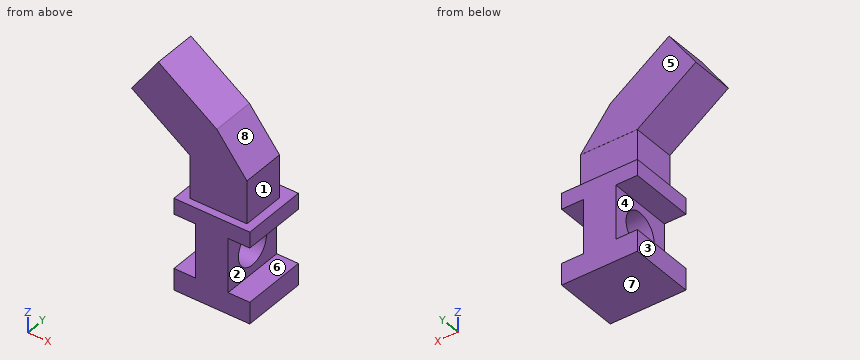
```python
from build123d import *

# Parameters (mm, degrees)
F1_DEPTH = 76.2
F2_R     = 21.9538330402
F3_DEPTH = 63.501
F4_W     = 66.6200816631
F4_H     = 50.9327836335
F5_DEPTH = 50.292
F7_DEPTH = 51.054
F9_DEPTH = 83.82


with BuildPart() as f1:
    # F0 (on Front) → F1 (new body)
    with BuildSketch(Plane.XZ):
        Polygon((-43.6762087762, -9.6735172633), (-43.6762087762, -35.0735172633), (45.2237912238, -35.0735172633), (45.2237912238, -9.6735172633), (19.8237912238, -9.6735172633), (19.8237912238, 53.8264827367), (45.2237912238, 53.8264827367), (45.2237912238, 72.5250117484), (-43.6762087762, 72.5250117484), (-43.6762087762, 53.8264827367), (-18.2762087762, 53.8264827367), (-18.2762087762, -9.6735172633), align=None)
    extrude(amount=F1_DEPTH)

    # F2 (on face) → F3 (cut, through all)
    with BuildSketch(Plane.YZ.offset(19.8237912238)):
        with Locations((-38.1, 22.0764827367)):
            Circle(F2_R)
    extrude(amount=-F3_DEPTH, mode=Mode.SUBTRACT)

    # F4 (on face) → F5 (join)
    with BuildSketch(Plane.XY.offset(72.5250117484)):
        with Locations((1.9566230476, -41.8805312365)):
            Rectangle(F4_W, F4_H)
    extrude(amount=F5_DEPTH)

    # F6 (on face) → F7 (join)
    with BuildSketch(Plane.XZ.offset(67.3469230533)):
        Polygon((0, 167.4694269896), (-31.353417784, 122.8170117484), (35.2666638792, 122.8170117484), align=None)
    extrude(amount=-F7_DEPTH)

    # F9 (add): a face of the model
    f9_faces = [f1.faces().sort_by_distance(p)[0] for p in [
        (-15.676708892, -41.8199230533, 145.143219369),
    ]]
    extrude(f9_faces, amount=F9_DEPTH)


solid = f1.part
```
Verification items for the finished model (mm, model axes). Face numbers are marked on the shaded views. A direction names the side the tool comes from. Coordinates: 2 decimals unless noted, no trailing zeros. Write each loop counter-clockwise with the first axis right and the second up, starting at its lowest first coordinate (ties: lowest second). Pieces come first, ordered by that corner, then holes. Notation, with made-up numbers: (41, 53) - (78, 53) arc R28 ccw to (78, 81) - close; hole circle Ø7 at (77, -6.5). An arc over 180 degrees is marked (long way). Write item = value, one per line.
Q1. Cross-section at D-D (y = -62.5). Enter the section's corners in (x, z), plus the area to 3 significant figures.
Answer:
outline = (-99.95, 170.98) - (-31.35, 122.82) - (-31.35, 72.53) - (-43.68, 72.53) - (-43.68, 53.83) - (-18.28, 53.83) - (-18.28, -9.67) - (-43.68, -9.67) - (-43.68, -35.07) - (45.22, -35.07) - (45.22, -9.67) - (19.82, -9.67) - (19.82, 53.83) - (45.22, 53.83) - (45.22, 72.53) - (35.27, 72.53) - (35.27, 122.82) - (0, 167.47) - (-68.6, 215.64) - close
area = 15,800 mm²
Q2. Cross-section at B-B (x = 16.5). Enter the section's corners in (y, z), plus the area to 3 significant figures.
Answer:
outline = (-76.2, -35.07) - (0, -35.07) - (0, 72.53) - (-16.41, 72.53) - (-16.41, 122.82) - (-16.29, 122.82) - (-16.29, 146.58) - (-67.35, 146.58) - (-67.35, 72.53) - (-76.2, 72.53) - close; hole circle Ø43.91 at (-38.1, 22.08)
area = 10,500 mm²
Q3. Go/stop test with flat-tipped pins: pin 1 Ø3 at (y, z) = (-52.5, 124) entering from +X; pin 2 Ø19 at (y, z) = (-46.5, 6.5) entering from -X; pin 3 Ø20.5 at (x, y) = (-30.5, -23.5) entering from +Z; pin 4 Ø8 at (x, z) = (4.5, -1.5) entering from +Y. Record where each tip stops, or that it passes through.
Answer:
pin_1 = 35.27
pin_2 = -18.28
pin_3 = 196.08
pin_4 = 0
Q4. Cross-section at C-C (z = 27.5). Enter the section's corners in (x, y), plus the area to 3 significant figures.
Answer:
outline = (-18.28, -76.2) - (19.82, -76.2) - (19.82, -59.37) - (-18.28, -59.37) - close; (-18.28, -16.83) - (19.82, -16.83) - (19.82, 0) - (-18.28, 0) - close
area = 1,280 mm²
Q5. Access from +Z, -Z, +X, -X, +Y, -Y to the whole of each face (thin tool, end or side, straight path). Record for the marked faces 1, 2, 3, 4 and 5.
Answer:
face_1 = +Z, +X, +Y, -Y
face_2 = +X, +Y, -Y
face_3 = -Z, -X, +Y, -Y
face_4 = -X, +Y, -Y
face_5 = +Z, +X, -X, +Y
Q6. Mould release check, pull along Z, two halves, no side actions. Record for the marked faces 6, 7 and 8: released by +Z, released by -Z, zero draft, split by the parting line, or undercut.
Answer:
face_6 = undercut
face_7 = released by -Z
face_8 = released by +Z
Q7. Material ranges on L1, parallel to Z at x = -35, y = -15; L2, parallel to Y at x = -52.5, z = 197; L3, parallel to Z at x = -11, y = -4.5, recorded low to high. Write a range as from..to.
Answer:
L1 = -35.07..-9.67, 53.83..72.53
L2 = -67.35..-16.29
L3 = -35.07..72.53
Q8. Cross-section at A-A (y = -38.1). Enter the section's corners in (x, z).
Answer:
outline = (-99.95, 170.98) - (-31.35, 122.82) - (-31.35, 72.53) - (-43.68, 72.53) - (-43.68, 53.83) - (-18.28, 53.83) - (-18.28, 44.03) - (19.82, 44.03) - (19.82, 53.83) - (45.22, 53.83) - (45.22, 72.53) - (35.27, 72.53) - (35.27, 122.82) - (0, 167.47) - (-68.6, 215.64) - close; (-43.68, -35.07) - (45.22, -35.07) - (45.22, -9.67) - (19.82, -9.67) - (19.82, 0.12) - (-18.28, 0.12) - (-18.28, -9.67) - (-43.68, -9.67) - close
